The listing builds one solid part. Answer for the finished solid, in the listing's coordinates (mm). Round coordinates to 2 decimals unless told otherwise and drop trailing zeros. Write each loop counter-clockwise with the first axis right and the second up, starting at its lowest first coordinate (ties: lowest second). Pieces come first, ordered by that corner, then holes. Notation, with made-up numbers: (23, 70) - (82, 70) arc R25 ccw to (82, 92) - close; hole circle Ø1 at (36, 2.25). An arc over 180 degrees is marked (long way). Answer as CSV lines item,"result". Start each with the question number.
Item 1: For a pull along Y with two mould halves and no side action, classify faces 1 (the flat face through (-2.5, 8, -163)), 2 (the cylindrical face through (-0.04, 48.37, -342.68)) as pulls with the +Y half, pulls with the -Y half, needs draft (parallel to the pull), parting line crosses it, or undercut.
Item 2: Straight lines are drawn through the part: line 1 along Z through (x, y) = (0.05, 50); line 2 along Y through (x, z) = (0.1, -350); line 3 along Z through (x, y) = (-2.2, 49). For each, find the intervals that lie inside material, in ascending order. Write a range as [from, to].
Item 3: A cutting plane is placed at B-B on z = -350. Determine the outline of the cut face in (x, y).
Item 4: Flat-ended cylindrical pins translate along their axes: pin 1 (9 mm diameter, centred on y = 0, z = 0, fed in from -X); pin 2 (19.5 mm diameter, centred on y = 50, z = -350, fed in from +X). Find the tip coordinate at first contact, or state that the pin passes through.
Item 5: A cutting plane is placed at A-A on y = 50. Determine the outline of the cut face in (x, z).
Autodesk Inventor part; units mm, degrees
ref_plane "YZ Plane" through (0, 0, 0) normal (1, 0, 0) x (0, 1, 0)
ref_plane "XZ Plane" through (0, 0, 0) normal (0, 1, 0) x (-1, 0, 0)
ref_plane "XY Plane" through (0, 0, 0) normal (0, 0, 1) x (1, 0, 0)
sketch "スケッチ1" plane through (0, 0, 0) normal (1, 0, 0) x (0, 1, 0)
  circle A0 centre (0, 0) radius 7.5
  circle A1 centre (50, -350) radius 7.5
  line L0 (81.3202, 54.372) -> (-63.1061, 54.372)
  line L1 (-63.1061, 54.372) -> (-63.1061, -385.952)
  line L2 (-63.1061, -385.952) -> (81.3202, -385.952)
  line L3 (81.3202, -385.952) -> (81.3202, 54.372)
  dimension "d0" = 50
  dimension "d1" = 350
  dimension "d2" = 15
  dimension "d3" = 15
extrude "押し出し1" add sketch "スケッチ1" along normal mid plane 5
properties part number "stay" material "鉄、可鍛鉄"
Geometry says:
1,face 1,"needs draft"
1,face 2,"undercut"
2,line 1,"z = [-385.95, -357.5], [-342.5, 54.37]"
2,line 2,"y = [-63.11, 42.5], [57.5, 81.32]"
2,line 3,"z = [-385.95, -357.43], [-342.57, 54.37]"
3,outline,"(-2.5, -63.11) - (2.5, -63.11) - (2.5, 42.5) - (-2.5, 42.5) - close; (-2.5, 57.5) - (2.5, 57.5) - (2.5, 81.32) - (-2.5, 81.32) - close"
4,pin 1,"passes through"
4,pin 2,"stops at x = 2.5"
5,outline,"(-2.5, -385.95) - (2.5, -385.95) - (2.5, -357.5) - (-2.5, -357.5) - close; (-2.5, -342.5) - (2.5, -342.5) - (2.5, 54.37) - (-2.5, 54.37) - close"
